Autodesk Inventor part; units mm, degrees
ref_plane "Work Plane1" through (10, 0, 0) normal (1, 0, 0) x (0, 1, 0)
ref_plane "XZ Plane" through (0, 0, 0) normal (0, 1, 0) x (-1, 0, 0)
ref_plane "XY Plane" through (0, 0, 0) normal (0, 0, 1) x (1, 0, 0)
sketch "Sketch1" plane through (0, 0, 0) normal (0, 1, 0) x (-1, 0, 0)
  circle A0 centre (0, 0) radius 10
  dimension "d0" = 20
extrude "Extrusion1" add sketch "Sketch1" along normal blind 220
ref_plane "Work Plane1" through (10, 0, 0) normal (1, 0, 0) x (0, 1, 0)
sketch "Sketch2" plane through (10, 0, 0) normal (1, 0, 0) x (0, 1, 0)
  line L0 (220, -10) -> (220, 10)
  line L1 (0, -10) -> (0, 10)
  line L2 (0, 0) -> (132.5, 0)
  circle A0 centre (132.5, 0) radius 1.25
  circle A1 centre (132.5, 0) radius 0.5
  circle A2 centre (132.5, 0.0309) radius 2.5
  line L3 (0, -10) -> (0, 10)
  line L4 (132.5, -2.4691) -> (0, -2.4691)
  line L5 (0, -2.4691) -> (0, 2.5309)
  line L6 (0, 2.5309) -> (132.5, 2.5309)
  line L7 (132.5, 2.5309) -> (132.5, -2.4691)
  line L8 (220, -10) -> (220, 10)
  line L9 (132.5, -2.4691) -> (220, -2.4691)
  line L10 (220, -2.4691) -> (220, 2.5309)
  line L11 (220, 2.5309) -> (132.5, 2.5309)
  line L12 (132.5, 2.5309) -> (132.5, -2.4691)
  dimension "d21" = 5
  dimension "d3" = 132.5
  dimension "d4" = 2.5
  dimension "d5" = 1
extrude "Extrusion2" cut sketch "Sketch2" against normal blind 0.5
sketch "Sketch3" plane through (9.5, 0, 0) normal (1, 0, 0) x (0, 0, -1)
  line L0 (2.4691, 0) -> (-2.5309, 0)
  circle A0 centre (-0.0309, 132.5) radius 0.75
  circle A1 centre (-0.0309, 132.5) radius 1.25
  line L1 (2.4691, 220) -> (2.4691, 0)
  line L2 (-2.5309, 220) -> (2.4691, 220)
  line L3 (-2.5309, 0) -> (-2.5309, 220)
  point P0 (0, 0)
  dimension "d24" = 1.5
  dimension "d25" = 2.5
extrude "Extrusion4" [suppressed]
chamfer "Chamfer5" [suppressed]
chamfer "Chamfer6" distance 0.5 angle 45 2 edges at (-9.9999, 220, -0.0319) (-9.9999, 0, -0.0319)
properties part number "wał_półkola" material "Stainless Steel"
Input: part model. Units: mm. Frame: model coordinates. Coordinates: 2 decimals unless noted, no trailing zeros. Loops run counter-clockwise (first coordinate to the right, second up) from the corner with the lowest first, then second, coordinate; pieces in that order, holes last. Notation, with made-up numbers: (66.25, -26.5) - (104.25, -26.5) arc R26 cw to (104.25, -0.5) - close; hole circle Ø11 at (89, -6). An arc over 180 degrees is marked (long way). Answer in a Markdown table with one row per item.
(1) Pin query (flat end, axial travel): P1, Ø5.5, axis at y = 141.5, z = 1, coming from the +X side; P2, Ø1, axis at y = 89, z = -1, coming from the +X side; P3, Ø8, axis at x = 7.5, y = 192, coming from the +Z side. Return the tip coordinate at first contact, or that it passes through.
Model answer:
| item | result |
|---|---|
| P1 | stops at x = 9.67 |
| P2 | stops at x = 9.5 |
| P3 | stops at z = 9.37 |
(2) Material intervals for L1, parallel to X at y = 155, z = -0.25; L2, parallel to Z at x = -0.5, y = 209; L3, parallel to X at y = 35.5, z = 3, sorted ascending. Write a range as from..to.
Model answer:
| item | result |
|---|---|
| L1 | x = -10..9.5 |
| L2 | z = -9.99..9.99 |
| L3 | x = -9.54..9.54 |
(3) Mould query, pull axis Z, two halves, no side actions, for faces 1 (the face through (9.5, 108, 0)), 2 (the face through (0, 220, 0)), 3 (the face through (-10, 108, 0)). Classes: pulls with the +Z half, pulls with the -Z half, needs draft (parallel to the pull), parting line crosses it, or undercut.
Model answer:
| item | result |
|---|---|
| face 1 | undercut |
| face 2 | needs draft |
| face 3 | parting line crosses it |
(4) Cut plane A-A on y = 58. Output: boundary loops of the cut face in (x, z).
Model answer:
| item | result |
|---|---|
| outline | (9.5, -2.47) - (9.5, 2.53) - (9.67, 2.53) arc R10 ccw (long way) to (9.69, -2.47) - close |
